Autodesk Fusion 360 part; units mm, degrees
sketch "Sketch1" plane through (0, 0, 0) normal (0, 0, 1) x (1, 0, 0)
  line L0 (0, 0) -> (254, 0) construction
  line L1 (0, 0) -> (-254, 0) construction
  circle A0 centre (-254, 0) radius 8.128
  circle A1 centre (254, 0) radius 8.128
  line L2 (0, 0) -> (0, 63.5) construction
  circle A2 centre (0, 63.5) radius 16.5
  line L3 (-254, -25.4) -> (0, 0)
  line L4 (0, 0) -> (251.46, -25.2727)
  arc A3 (-254, 25.4) -> (-248.9703, -24.897) centre (-254, 0) ccw
  arc A4 (251.46, -25.2727) -> (258.9348, 24.916) centre (254, 0) ccw
  line L5 (-0.0285, 88.9) -> (-254, 25.4)
  line L6 (-0.0285, 88.9) -> (258.9348, 24.916)
  arc A5 (11.8546, 85.9639) -> (-11.9289, 85.9245) centre (0, 63.5) ccw
  dimension "d1" = 254
  dimension "d2" = 254
  dimension "d3" = 16.256
  dimension "d4" = 16.256
  dimension "d5" = 33
extrude "Extrude1" add sketch "Sketch1" along normal blind 24.2 contours L3 L4 A3 A4 L5 L6
fillet "Fillet1" radius 76.2 2 edges at (0, 0, 12.1) (-0.0285, 88.9, 12.1)
fillet "Fillet2" radius 3.81 16 edges at (-130.8006, -13.0801, 24.2) (-0.0001, -0.382, 24.2) (129.5305, -13.0183, 24.2) (279.1229, -3.7416, 24.2) (-279.4, 0, 24.2) (-130.8006, -13.0801, 0) (-0.0001, -0.382, 0) (129.5305, -13.0183, 0) (279.1229, -3.7416, 0) (-279.4, 0, 0) (138.6465, 54.6365, 24.2) (-0.0253, 86.5815, 24.2) (-136.2013, 54.853, 24.2) (-136.2013, 54.853, 0) (-0.0253, 86.5815, 0) (138.6465, 54.6365, 0)
scale "Scale1" factor 0.5 about (-16.5, 63.5, 24.2) bodies 1
sketch "Sketch2" plane through (0, 0, 24.2) normal (0, 0, 1) x (-1, 0, 0)
  circle A0 centre (8.25, -63.5) radius 8.25
  circle A1 centre (-118.75, -31.75) radius 4.064
  circle A2 centre (135.25, -31.75) radius 4.064
  line L0 (135.3412, -20.9554) -> (12.2402, -33.2655)
  arc A3 (4.259, -33.2635) -> (12.2402, -33.2655) centre (8.2595, 6.541) ccw
  line L1 (4.259, -33.2635) -> (-117.6705, -21.0091)
  arc A4 (-117.6705, -21.0091) -> (-120.8054, -42.3475) centre (-118.75, -31.75) ccw
  line L2 (-120.8054, -42.3475) -> (-0.4722, -72.0791)
  arc A5 (-0.4722, -72.0791) -> (16.9892, -72.0549) centre (8.2097, -36.9408) ccw
  line L3 (16.9892, -72.0549) -> (135.0248, -42.5427)
  arc A6 (135.0248, -42.5427) -> (135.3412, -20.9554) centre (135.25, -31.75) ccw
  circle A7 centre (8.25, -63.5) radius 10.25
  dimension "d13" = 20.5
extrude "Extrude2" cut sketch "Sketch2" against normal blind 2.1 contours A5 A7 | A5 A7
For this review, take the finished solid that the model builds, in its own axes (mm). A direction names the side the tool comes from. Round coordinates to 2 decimals unless told otherwise and drop trailing zeros.
Q1. To check wall thickness, follow line 1 along Y through (x, z) = (-8.25, 22.6); line 2 along Y through (x, z) = (-8.25, 19.75); line 3 along Z through (x, y) = (-52.5, 63.5). State the ranges of each line that lie inside material, in increasing order.
Result sheet:
line 1: y = 31.58 to 53.25, 73.75 to 75.02
line 2: y = 31.56 to 55.25, 71.75 to 75.04
line 3: z = 12.13 to 24.17
Q2. Add section A-A on z = 17.5. Give the number of separate pieces and of enclosed holes in the cut face, plus the area to 3 significant figures.
Result sheet:
separate pieces: 1
enclosed holes: 3
area: 9,080 mm2
Q3. Machinability: for faces 5 (the face through (-72.84, 25.87, 23.66)), 6 (the face through (-74.513, 25.124, 18.092)), 7 (the face through (-74.57, 25.694, 12.643)), 8 (the face through (-12.98, 72.594, 23.165)), which of the approach directions +Z, -Z, +X, -X, +Y, -Y give a long, thin tool a straight path to every point of the face, cutting with its end or side? Answer none if there is none.
Result sheet:
face 5: +Z, -Y
face 6: +Z, -Z, -Y
face 7: -Z, -Y
face 8: +Z
Q4. Mouldability with a two-part tool opening along Y and no side actions: class faces 1 (the face through (57.43, 25.73, 23.66)), 2 (the face through (61.78, 58.3, 12.64)), 3 (the face through (-139.31, 31.57, 18.07)), 4 (the face through (-9.32, 55.32, 17.03)) as +Y half, -Y half, draft (parallel to the pull), parting line (faces both ways), or undercut.
Result sheet:
face 1: -Y half
face 2: +Y half
face 3: undercut
face 4: undercut
Q5. Insertion check: pin 1 Ø5 at (x, z) = (62.5, 15) entering from -Y; pin 2 Ø6.5 at (x, y) = (-135.25, 31.75) entering from -Z. Each pin has a flat end and moves straight along its axis. Give the tip position at first contact, or say it passes through.
Result sheet:
pin 1: stops at y = 24.39
pin 2: passes through
